```python
from build123d import *
from OCP.BRepFilletAPI import BRepFilletAPI_MakeChamfer

# Parameters (mm, degrees)
SKETCH1_W           = 40
SKETCH1_H           = 80
BOSS_EXTRUDE1_DEPTH = 6
SKETCH2_R           = 5
BOSS_EXTRUDE2_DEPTH = 15
CHAMFER1_SIZE       = 5
CHAMFER1_SIZE2      = 0.881634904


with BuildPart() as part:
    # Sketch1 → Boss-Extrude1 (new, symmetric)
    with BuildSketch(Plane(origin=(0, 0, 0), x_dir=(1, 0, 0), z_dir=(0, 1, 0))):
        Rectangle(SKETCH1_W, SKETCH1_H)
    extrude(amount=BOSS_EXTRUDE1_DEPTH, both=True)

    # Sketch2 → Boss-Extrude2 (add)
    with BuildSketch(Plane(origin=(0, 0, -40), x_dir=(-1, 0, 0), z_dir=(0, 0, -1))):
        with Locations(Location((13, 0, 0), (0, 0, 180))):
            Circle(SKETCH2_R)
        with Locations(Location((-13, 0, 0), (0, 0, 180))):
            Circle(SKETCH2_R)
    extrude(amount=BOSS_EXTRUDE2_DEPTH)

    # Chamfer1: one chamfer whose edges measure the first distance from different faces: ONE call of the kernel's chamfer builder (chamfer() names one face for all edges)
    chamfer1_edges_1 = [part.edges().sort_by_distance(p)[0] for p in [
        (-18, 0, -55),
    ]]
    chamfer1_side_1 = [part.faces().sort_by_distance(p)[0] for p in [
        (-18, 0, -47.5),
    ]]
    chamfer1_edges_2 = [part.edges().sort_by_distance(p)[0] for p in [
        (8, 0, -55),
    ]]
    chamfer1_side_2 = [part.faces().sort_by_distance(p)[0] for p in [
        (8, 0, -47.5),
    ]]
    chamfer1 = BRepFilletAPI_MakeChamfer(part.part.solid().wrapped)
    for e in chamfer1_edges_1:
        chamfer1.Add(CHAMFER1_SIZE, CHAMFER1_SIZE2, e.wrapped, chamfer1_side_1[0].wrapped)  # the first distance lies on this face
    for e in chamfer1_edges_2:
        chamfer1.Add(CHAMFER1_SIZE, CHAMFER1_SIZE2, e.wrapped, chamfer1_side_2[0].wrapped)  # the first distance lies on this face
    add(Compound.cast(chamfer1.Shape()), mode=Mode.REPLACE)


solid = part.part
```
Input: part model. Units: mm. Frame: model coordinates. A direction names the side the tool comes from. Give positions to 0.01 mm unless a question says otherwise; leave off trailing zeros. Order: outer loops, then holes, each group sorted by start corner. A loop starts at its lowest first (then second) coordinate and runs counter-clockwise, first axis right, second up. Notation, with made-up numbers: (42, 76.5) - (56, 76.5) arc R22 ccw to (56, 111.5) - close; hole circle Ø8 at (-16, 28). An arc over 180 degrees is marked (long way). One line per item, written item: value.
1. Line query: probe 1 along Z at (x, y) = (-5, -4.25); probe 2 along X at (y, z) = (-4, -41.5); probe 3 along Y at (x, z) = (-8.5, -50). Output: solid intervals per line, ascending.
Determined:
probe 1: -40 to 40
probe 2: -16 to -10, 10 to 16
probe 3: -2.18 to 2.18
2. Cut plane A-A, the plane x = -13. Output: boundary loops of the cut face in (y, z), and give its area (3 significant figures).
Determined:
outline: (-6, -40) - (-5, -40) - (-5, -50) - (-4.12, -55) - (4.12, -55) - (5, -50) - (5, -40) - (6, -40) - (6, 40) - (-6, 40) - close
area: 1,110 mm2
3. Draft query along X for faces 1 (the face through (-13, 0, -55)), 2 (the face through (17.77, -1.5, -44.93)), 3 (the face through (20, 0, 1)), 4 (the face through (-20, 0, 1)). Return one class per face: released by +X, released by -X, zero draft, split by the parting line, or undercut.
Determined:
face 1: zero draft
face 2: undercut
face 3: released by +X
face 4: released by -X
4. Cut plane C-C, the plane x = -3. Output: boundary loops of the cut face in (y, z).
Determined:
outline: (-6, -40) - (6, -40) - (6, 40) - (-6, 40) - close
5. Reachability of faces 5 (the face through (0, 0, -40)), 6 (the face through (0, 0, 40)) from +Z, -Z, +X, -X, +Y, -Y: full face, straight path, thin tool, end or side. Return the list, or none.
Determined:
face 5: -Z
face 6: +Z, +X, -X, +Y, -Y
6. Cut plane B-B, the plane y = 0. Output: boundary loops of the cut face in (x, z).
Determined:
outline: (-20, -40) - (-18, -40) - (-18, -50) - (-17.12, -55) - (-8.88, -55) - (-8, -50) - (-8, -40) - (8, -40) - (8, -50) - (8.88, -55) - (17.12, -55) - (18, -50) - (18, -40) - (20, -40) - (20, 40) - (-20, 40) - close
